from build123d import *

# Parameters (mm, degrees)
SKETCH054_W          = 53.7
SKETCH054_H          = 59.2
SKETCH054_R          = 1.75
PAD015_DEPTH         = 1.6
SKETCH055_W          = 53.7
SKETCH055_H          = 55.7
SKETCH055_W_2        = 50.5
SKETCH055_H_2        = 52.5
PAD016_DEPTH         = 40
CHAMFER002_SIZE      = 1.15
FILLET006_R          = 1
SKETCH056_W          = 5
SKETCH056_H          = 3
SKETCH056_W_2        = 5.25
SKETCH056_H_2        = 2.5
POCKET016_DEPTH      = 27.851
POCKET016_DEPTH_BACK = 31.351
POCKET017_DEPTH      = 31.351
POCKET022_DEPTH      = 27.851
SKETCH058_W          = 9
SKETCH058_H          = 4
POCKET018_DEPTH      = 26.851
POCKET018_DEPTH_BACK = 26.851
SKETCH059_R          = 3.2
PAD017_DEPTH         = 2.2
SKETCH060_R          = 1.75
POCKET019_DEPTH      = 3.801
SKETCH061_W          = 1.5
SKETCH061_H          = 0.4
POCKET020_DEPTH      = 8


with BuildPart() as part:
    # Sketch054 → Pad015 (new body)
    with BuildSketch(Plane.XY):
        with Locations((0, -1.75)):
            Rectangle(SKETCH054_W, SKETCH054_H)
        with Locations((0, 19.652)):
            Circle(SKETCH054_R, mode=Mode.SUBTRACT)
    extrude(amount=PAD015_DEPTH)

    # Sketch055 → Pad016 (join)
    with BuildSketch(Plane.XY.offset(1.6)):
        Rectangle(SKETCH055_W, SKETCH055_H)
        Rectangle(SKETCH055_W_2, SKETCH055_H_2, mode=Mode.SUBTRACT)
    extrude(amount=PAD016_DEPTH)

    # Chamfer002
    chamfer002_edges = [part.edges().sort_by_distance(p)[0] for p in [
        (0, 26.25, 41.6),
        (0, -26.25, 41.6),
    ]]
    chamfer(chamfer002_edges, length=CHAMFER002_SIZE)

    # Fillet006
    fillet006_edges = [part.edges().sort_by_distance(p)[0] for p in [
        (-25.25, -26.25, 21.025),
        (-26.85, -27.85, 21.6),
        (-25.25, 26.25, 21.025),
        (-26.85, 27.85, 21.6),
        (25.25, 26.25, 21.025),
        (26.85, 27.85, 21.6),
        (25.25, -26.25, 21.025),
        (26.85, -27.85, 21.6),
        (-26.85, -31.35, 0.8),
        (26.85, -31.35, 0.8),
    ]]
    fillet(fillet006_edges, radius=FILLET006_R)

    # Sketch056 → Pocket016 (cut, two sides)
    with BuildSketch(Plane.XZ) as pocket016_sk:
        with Locations((-15, 36.1)):
            Rectangle(SKETCH056_W, SKETCH056_H)
        with Locations((15, 36.1)):
            Rectangle(SKETCH056_W, SKETCH056_H)
        with Locations((-9.125, 40.35)):
            Rectangle(SKETCH056_W_2, SKETCH056_H_2)
        with Locations((9.125, 40.35)):
            Rectangle(SKETCH056_W_2, SKETCH056_H_2)
    extrude(amount=-POCKET016_DEPTH, mode=Mode.SUBTRACT)
    extrude(pocket016_sk.sketch, amount=POCKET016_DEPTH_BACK, mode=Mode.SUBTRACT)

    # Sketch057 → Pocket017 (cut, through all)
    with BuildSketch(Plane.XZ):
        with BuildLine():
            Line((23.733, 17.8), (23.733, 1.6))
            Line((23.733, 1.6), (-23.733, 1.6))
            Line((-23.733, 1.6), (-23.733, 17.8))
            ThreePointArc((-18.733, 22.8), (-22.268534, 21.335534), (-23.733, 17.8))
            Line((-18.733, 22.8), (18.733, 22.8))
            ThreePointArc((23.733, 17.8), (22.268534, 21.335534), (18.733, 22.8))
        make_face()
    extrude(amount=POCKET017_DEPTH, mode=Mode.SUBTRACT)

    # Sketch063 → Pocket022 (cut, through all)
    with BuildSketch(Plane.XZ):
        with BuildLine():
            Line((-22.733, 18.6), (-15.733, 18.6))
            ThreePointArc((-14.733, 17.599995), (-15.025892, 18.307105), (-15.733, 18.6))
            Line((-14.733, 17.599995), (-14.733034, 10.599995))
            ThreePointArc((-15.733034, 9.6), (-15.025929, 9.892892), (-14.733034, 10.599995))
            Line((-15.733034, 9.6), (-22.733, 9.6))
            ThreePointArc((-23.733, 10.6), (-23.440107, 9.892893), (-22.733, 9.6))
            Line((-23.733, 10.6), (-23.733, 17.6))
            ThreePointArc((-22.733, 18.6), (-23.440107, 18.307107), (-23.733, 17.6))
        make_face()
        with BuildLine():
            Line((15.733, 18.599966), (22.733, 18.599966))
            ThreePointArc((23.733, 17.599966), (23.440107, 18.307073), (22.733, 18.599966))
            Line((23.733, 17.599966), (23.733, 10.6))
            ThreePointArc((22.733, 9.6), (23.440107, 9.892893), (23.733, 10.6))
            Line((22.733, 9.6), (15.733, 9.6))
            ThreePointArc((14.733, 10.6), (15.025893, 9.892893), (15.733, 9.6))
            Line((14.733, 10.6), (14.733, 17.599966))
            ThreePointArc((15.733, 18.599966), (15.025893, 18.307073), (14.733, 17.599966))
        make_face()
    extrude(amount=-POCKET022_DEPTH, mode=Mode.SUBTRACT)

    # Sketch058 → Pocket018 (cut, two sides)
    with BuildSketch(Plane.YZ) as pocket018_sk:
        with Locations((-16, 39.6)):
            Rectangle(SKETCH058_W, SKETCH058_H)
        with Locations((16, 39.6)):
            Rectangle(SKETCH058_W, SKETCH058_H)
    extrude(amount=-POCKET018_DEPTH, mode=Mode.SUBTRACT)
    extrude(pocket018_sk.sketch, amount=POCKET018_DEPTH_BACK, mode=Mode.SUBTRACT)

    # Sketch059 → Pad017 (join)
    with BuildSketch(Plane.XY.offset(1.6)):
        with Locations((-15.621, -15.348)):
            Circle(SKETCH059_R)
        with Locations((19.431, -15.348)):
            Circle(SKETCH059_R)
        with Locations((19.431, -28.048)):
            Circle(SKETCH059_R)
        with Locations((-15.621, -28.048)):
            Circle(SKETCH059_R)
    extrude(amount=PAD017_DEPTH)

    # Sketch060 → Pocket019 (cut, through all)
    with BuildSketch(Plane.XY.offset(3.8)):
        with Locations((-15.621, -15.348)):
            Circle(SKETCH060_R)
        with Locations((19.431, -15.348)):
            Circle(SKETCH060_R)
        with Locations((19.431, -28.048)):
            Circle(SKETCH060_R)
        with Locations((-15.621, -28.048)):
            Circle(SKETCH060_R)
    extrude(amount=-POCKET019_DEPTH, mode=Mode.SUBTRACT)

    # Sketch061 → Pocket020 (cut)
    with BuildSketch(Plane.XY.offset(41.6)):
        with Locations((-21.5, 26.45)):
            Rectangle(SKETCH061_W, SKETCH061_H)
        with Locations((21.5, 26.45)):
            Rectangle(SKETCH061_W, SKETCH061_H)
        with Locations((21.5, -26.45)):
            Rectangle(SKETCH061_W, SKETCH061_H)
        with Locations((-21.5, -26.45)):
            Rectangle(SKETCH061_W, SKETCH061_H)
    extrude(amount=-POCKET020_DEPTH, mode=Mode.SUBTRACT)


solid = part.part
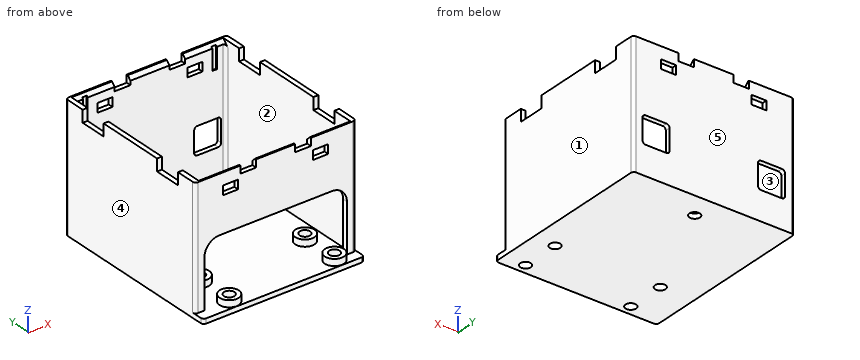
Model file for the job. Use its own axes, mm. Face numbers are marked on the shaded views. A direction names the side the tool comes from. Give positions to 0.01 mm unless a question says otherwise; leave off trailing zeros. Order: outer loops, then holes, each group sorted by start corner. A loop starts at its lowest first (then second) coordinate and runs counter-clockwise, first axis right, second up. Notation, with made-up numbers: (-26, 61) - (9, 61) arc R27 ccw to (9, 90) - close; hole circle Ø9 at (15.5, 43.5). An arc over 180 degrees is marked (long way). Return JSON: item names as keys, results as strings.
1) Pull direction X, two halves, no side cores. Call the marked faces 3, 4 and 5: pulls with the +X half, pulls with the -X half, needs draft (parallel to the pull), parting line crosses it, or undercut.
Geometry says:
{"face 3": "undercut", "face 4": "pulls with the -X half", "face 5": "needs draft"}
2) Probe line 1 (X direction, y = -21.5, z = 23); line 2 (Y direction, x = 0, z = 0.9); line 3 (Y direction, x = -9, z = 37). List the from-to ranges inside material, lowest first. Write a range as from..to.
Geometry says:
{"line 1": "-26.85..-25.25, 25.25..26.85", "line 2": "-31.35..17.9, 21.4..27.85", "line 3": "-27.85..-26.25, 26.25..27.85"}
3) Cut at B-B, the plane y = 0.5. Give the cut face in (x, z).
Geometry says:
{"outline": "(-26.85, 0) - (26.85, 0) - (26.85, 41.6) - (25.25, 41.6) - (25.25, 1.6) - (-25.25, 1.6) - (-25.25, 41.6) - (-26.85, 41.6) - close"}
4) Flat gauge pins, fed straight in: P1, Ø1.8, axis at x = -26, z = 39, coming from the -Y side; P2, Ø8, axis at x = 0.5, y = -21, coming from the +Z side. Where does each tip first touch, or does it go through?
Geometry says:
{"P1": "y = -27.85", "P2": "z = 1.6"}
5) 3-axis set-ups, long thin cutter, end or side, ignore diameter. For the marked faces 1 and 2: which of +Z, -Z, +X, -X, +Y, -Y reach the whole face in a straight line?
Geometry says:
{"face 1": "+Z, -Z, +X, +Y, -Y", "face 2": "+Z"}
6) Cut at C-C, the plane z = 21. Give the cut face in (x, y).
Geometry says:
{"outline": "(-26.85, -26.85) arc R1 ccw to (-25.85, -27.85) - (-22.57, -27.85) - (-22.57, -26.25) - (-24.25, -26.25) arc R1 cw to (-25.25, -25.25) - (-25.25, 25.25) arc R1 cw to (-24.25, 26.25) - (24.25, 26.25) arc R1 cw to (25.25, 25.25) - (25.25, -25.25) arc R1 cw to (24.25, -26.25) - (22.57, -26.25) - (22.57, -27.85) - (25.85, -27.85) arc R1 ccw to (26.85, -26.85) - (26.85, 26.85) arc R1 ccw to (25.85, 27.85) - (-25.85, 27.85) arc R1 ccw to (-26.85, 26.85) - close"}
7) Cut at A-A, the plane x = 0. Give the cut face in (y, z), plus the area to 3 significant figures.
Geometry says:
{"outline": "(-31.35, 0) - (17.9, 0) - (17.9, 1.6) - (-31.35, 1.6) - close; (-27.85, 22.8) - (-26.25, 22.8) - (-26.25, 40.45) - (-27.4, 41.6) - (-27.85, 41.6) - close; (21.4, 0) - (27.85, 0) - (27.85, 41.6) - (27.4, 41.6) - (26.25, 40.45) - (26.25, 1.6) - (21.4, 1.6) - close", "area": "182 mm²"}
